```python
from build123d import *

# Parameters (mm, degrees)
SKETCH1_R           = 115
BOSS_EXTRUDE1_DEPTH = 50
SKETCH2_R           = 10
SKETCH3_R           = 25
CUT_EXTRUDE1_DEPTH  = 171.146995272


with BuildPart() as part:
    # Sketch1 → Boss-Extrude1 (new body)
    with BuildSketch(Plane.XY):
        Circle(SKETCH1_R)
    extrude(amount=BOSS_EXTRUDE1_DEPTH)

    # Sketch2 → Cut-Revolve1 (revolve, cut)
    with BuildSketch(Plane(origin=(0, 0, 0), x_dir=(0, 0, -1), z_dir=(1, 0, 0)), mode=Mode.PRIVATE) as cut_revolve1_sk:
        with Locations((-25, 115)):
            Circle(SKETCH2_R)
    revolve(cut_revolve1_sk.sketch.rotate(Axis((0, 0, 0), (0, 0, 1)), 90), axis=Axis((0, 0, 0), (0, 0, 1)), mode=Mode.SUBTRACT)

    # Sketch3 → Cut-Extrude1 (cut, through all)
    with BuildSketch(Plane(origin=(0, 0, 0), x_dir=(-1, 0, 0), z_dir=(0, 0, -1))):
        Circle(SKETCH3_R)
    extrude(amount=-CUT_EXTRUDE1_DEPTH, mode=Mode.SUBTRACT)


solid = part.part
```
The listing builds one solid part. Answer for the finished solid, in the listing's coordinates (mm). Coordinates: 2 decimals unless noted, no trailing zeros. Loops run counter-clockwise (first coordinate to the right, second up) from the corner with the lowest first, then second, coordinate; pieces in that order, holes last. Notation, with made-up numbers: (-19.5, 74.25) -> (-3.5, 74.25) arc R18 ccw to (-3.5, 108.25) -> close; hole circle Ø10 at (23.25, 78). An arc over 180 degrees is marked (long way). Use one line per item in the form item = value. Start each with the question number.
Item 1: Consider L1, parallel to Y at x = 0, z = 13; L2, parallel to X at y = 14, z = 11; L3, parallel to X at y = 12, z = 26.5. Determine where each line is inside the solid, lowest interval first. Write a range as [from, to].
Item 2: Flat-ended cylindrical pins translate along their axes: pin 1 Ø4 at (y, z) = (11, 33.5) entering from -X; pin 2 Ø5 at (y, z) = (-48, 34.5) entering from -X; pin 3 Ø10 at (x, z) = (47, 11) entering from -Y. Find the tip coordinate at first contact, or state that the pin passes through.
Item 3: The part is cut by section A-A on y = 0. Determine the outline of the cut face in (x, z).
Item 4: The part is cut by section C-C on z = 45. Determine the outline of the cut face in (x, y), then the cut area to 3 significant figures.
Item 5: The mould has two halves that part along X. Classify faces 1 (the face through (-2, 27, 50)), 2 (the face through (-24.93, -112.265, 7.395)), 3 (the face through (-23.846, 7.509, 24.65)): released by +X, released by -X, zero draft, split by the parting line, or undercut.
Answer key:
q1.L1 = [-115, -25], [25, 115]
q1.L2 = [-114.14, -20.71], [20.71, 114.14]
q1.L3 = [-104.43, -21.93], [21.93, 104.43]
q2.pin_1 = -114.59
q2.pin_2 = -105.59
q2.pin_3 = -107.06
q3.outline = (-115, 0) -> (-25, 0) -> (-25, 50) -> (-115, 50) -> (-115, 35) arc R10 cw to (-115, 15) -> close; (25, 0) -> (115, 0) -> (115, 15) arc R10 cw to (115, 35) -> (115, 50) -> (25, 50) -> close
q4.outline = circle Ø230 at (0, 0); hole circle Ø50 at (0, 0)
q4.area = 39,600 mm2
q5.face_1 = zero draft
q5.face_2 = split by the parting line
q5.face_3 = undercut
